Autodesk Fusion 360 part; units mm, degrees
sketch "Sketch1" plane through (0, 0, 0) normal (0, 1, 0) x (1, 0, 0)
  line L0 (0, 0) -> (431.8, 0)
  line L1 (215.9, 160.6296) -> (152.4, 160.6296)
  line L2 (215.9, 160.6296) -> (279.4, 160.6296)
  line L3 (279.4, 160.6296) -> (431.8, 0)
  line L4 (152.4, 160.6296) -> (0, 0)
  circle A0 centre (247.65, 132.6896) radius 1.905
  circle A1 centre (184.15, 150.4696) radius 1.905
  circle A2 centre (317.8261, 101.6767) radius 1.905
  circle A3 centre (374.9476, 41.4706) radius 1.905
  circle A4 centre (247.65, 150.4696) radius 1.905
  circle A5 centre (184.15, 132.6896) radius 1.905
  circle A6 centre (292.4768, 128.3949) radius 1.905
  circle A7 centre (400.2969, 14.7524) radius 1.905
  dimension "d1" = 431.8
  dimension "d3" = 63.5
  dimension "d4" = 63.5
extrude "Extrude3" add sketch "Sketch1" along normal blind 2.794
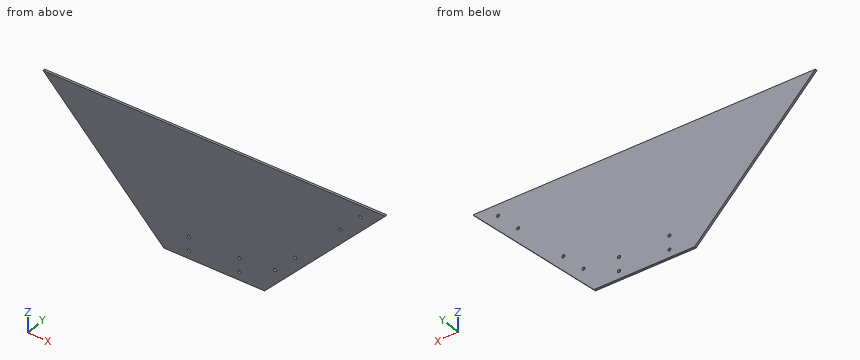
Model file for the job. Use its own axes, mm. Round coordinates to 2 decimals unless told otherwise and drop trailing zeros. Loops run counter-clockwise (first coordinate to the right, second up) from the corner with the lowest first, then second, coordinate; pieces in that order, holes last. Notation, with made-up numbers: (-25, -20) -> (-13, -20) arc R8 cw to (-13, -15) -> close; hole circle Ø8 at (84.5, 9.25). An arc over 180 degrees is marked (long way). Answer as CSV lines item,"result". Start each with the question number.
1) Slice it at A-A (y = 1.35). State how many separate pieces and enclosed holes the cut face has, plus the area to 3 significant figures.
2) Slice it at B-B (x = 72.5). List the corners of the cut face in (y, z) (3 decimals).
3) Pin check, flat tips, straight feed: P1, Ø1.5, axis at y = 2, z = -93, coming from the +X side; P2, Ø3, axis at x = 247.65, z = -150.47, coming from the -Y side. Stop position of each tip, or through.
4) Slice it at C-C (z = -67.5). List the corners of the cut face in (x, y), plus the area to 3 significant figures.
5) Probe line 1 along Z through (x, y) = (184.15, 1.9); line 2 along X through (y, z) = (2.45, -100.5); line 3 along X through (y, z) = (1.25, -127). List the from-to ranges inside material, lowest first.
Filled in:
1,separate pieces,"1"
1,enclosed holes,"8"
1,area,"44,800 mm2"
2,outline,"(0, -76.415) -> (2.794, -76.415) -> (2.794, 0) -> (0, 0) -> close"
3,P1,"stops at x = 344.28"
3,P2,"passes through"
4,outline,"(64.04, 0) -> (367.76, 0) -> (367.76, 2.79) -> (64.04, 2.79) -> close"
4,area,"849 mm2"
5,line 1,"z = -160.63 to -152.37, -148.56 to -134.59, -130.78 to 0"
5,line 2,"x = 95.35 to 316.33, 319.32 to 336.45"
5,line 3,"x = 120.49 to 291.18, 293.77 to 311.31"
